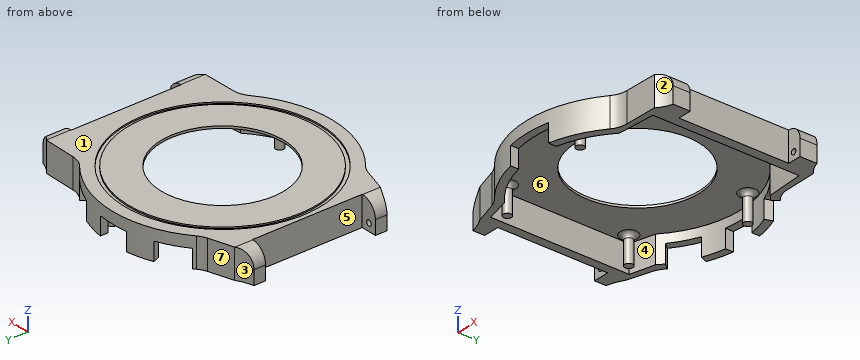
```python
from build123d import *

# Parameters (mm, degrees)
PAD_DEPTH       = 6.5
POCKET_DEPTH    = 6
SKETCH002_R     = 13.5
POCKET001_DEPTH = 1
SKETCH003_W     = 5.4
SKETCH003_H     = 6.5
PAD001_DEPTH    = 3
POCKET002_DEPTH = 10
SKETCH008_R     = 0.6
POCKET003_DEPTH = 2
SKETCH009_R     = 0.6
POCKET004_DEPTH = 2
FILLET_R        = 2.9
FILLET001_R     = 2.9
FILLET002_R     = 5
FILLET003_R     = 5
FILLET004_R     = 5
FILLET005_R     = 5
SKETCH010_W     = 3.95
SKETCH010_H     = 6.5
PAD002_DEPTH    = 3.5
POCKET005_DEPTH = 10
SKETCH012_R     = 0.6
POCKET006_DEPTH = 2
SKETCH013_R     = 0.6
POCKET007_DEPTH = 2
FILLET006_R     = 3.4
FILLET007_R     = 3.4
SKETCH014_R     = 21.6
SKETCH014_R_2   = 20.8
POCKET008_DEPTH = 0.3
SKETCH015_R     = 0.9
PAD003_DEPTH    = 6
FILLET008_R     = 1
POCKET009_DEPTH = 4
POCKET010_DEPTH = 4


with BuildPart() as part:
    # Sketch → Pad (new body)
    with BuildSketch(Plane.XY):
        with BuildLine():
            Line((-22.5019915649, 16), (-22.5019915649, -16))
            Line((-22.5019915649, -16), (-16.2858834578, -17.9))
            ThreePointArc((-16.2858834578, -17.9), (0.2206895736, -24.1989937004), (16.6096357576, -17.6))
            Line((16.6096357576, -17.6), (25.6083856708, -17.45))
            Line((25.6083856708, 17.45), (25.6083856708, -17.45))
            Line((16.6096357576, 17.6), (25.6083856708, 17.45))
            ThreePointArc((16.6096357576, 17.6), (0.2206895736, 24.1989937004), (-16.2858834578, 17.9))
            Line((-22.5019915649, 16), (-16.2858834578, 17.9))
        make_face()
    extrude(amount=PAD_DEPTH)

    # Sketch001 → Pocket (cut)
    with BuildSketch(Plane.XY):
        with BuildLine():
            Line((-15.2429491897, 16.55), (-20.5746937447, 15.2))
            Line((-20.5746937447, 15.2), (-20.5746937447, -15.2))
            Line((-20.5746937447, -15.2), (-15.2429491897, -16.55))
            ThreePointArc((-15.2429491897, -16.55), (0, -22.5), (15.2429491897, -16.55))
            Line((15.2429491897, -16.55), (23.5278752606, -16.05))
            Line((23.5278752606, 16.05), (23.5278752606, -16.05))
            Line((15.2429491897, 16.55), (23.5278752606, 16.05))
            ThreePointArc((15.2429491897, 16.55), (0, 22.5), (-15.2429491897, 16.55))
        make_face()
    extrude(amount=POCKET_DEPTH, mode=Mode.SUBTRACT)

    # Sketch002 (on Face19 of Pocket) → Pocket001 (cut)
    with BuildSketch(Plane(origin=(0, 0, 6), x_dir=(1, 0, 0), z_dir=(0, 0, -1))):
        Circle(SKETCH002_R)
    extrude(amount=-POCKET001_DEPTH, mode=Mode.SUBTRACT)

    # Sketch003 (on Face6 of Pocket001) → Pad001 (join)
    with BuildSketch(Plane.YZ.offset(25.6083856708)):
        with Locations((-14.75, 3.25)):
            Rectangle(SKETCH003_W, SKETCH003_H)
        with Locations((14.75, 3.25)):
            Rectangle(SKETCH003_W, SKETCH003_H)
    extrude(amount=PAD001_DEPTH)

    # Sketch006 → Pocket002 (cut)
    with BuildSketch(Plane.XY.offset(6.5)):
        with BuildLine():
            ThreePointArc((25.6083856708, 17.45), (27.0135397777, 16.4426436477), (28.6083856708, 15.775042373))
            Line((28.6083856708, 17.45), (28.6083856708, 15.775042373))
            Line((28.6083856708, 17.45), (25.6083856708, 17.45))
        make_face()
        with BuildLine():
            ThreePointArc((28.6083856708, -15.775042373), (27.0135397777, -16.4426436477), (25.6083856708, -17.45))
            Line((28.6083856708, -17.45), (25.6083856708, -17.45))
            Line((28.6083856708, -15.775042373), (28.6083856708, -17.45))
        make_face()
    extrude(amount=-POCKET002_DEPTH, mode=Mode.SUBTRACT)

    # Sketch008 (on Face27 of Pocket002) → Pocket003 (cut)
    with BuildSketch(Plane(origin=(0, -12.05, 0), x_dir=(-1, 0, 0), z_dir=(0, 1, 0))):
        with Locations((-26.9083856708, 1.7)):
            Circle(SKETCH008_R)
    extrude(amount=-POCKET003_DEPTH, mode=Mode.SUBTRACT)

    # Sketch009 (on Face26 of Pocket003) → Pocket004 (cut)
    with BuildSketch(Plane.XZ.offset(-12.05)):
        with Locations((26.9083856708, 1.7)):
            Circle(SKETCH009_R)
    extrude(amount=-POCKET004_DEPTH, mode=Mode.SUBTRACT)

    # Fillet
    fillet_edges = [part.edges().sort_by_distance(p)[0] for p in [
        (28.608386, -13.912521, 6.5),
    ]]
    fillet(fillet_edges, radius=FILLET_R)

    # Fillet001
    fillet001_edges = [part.edges().sort_by_distance(p)[0] for p in [
        (28.608386, 13.912521, 6.5),
    ]]
    fillet(fillet001_edges, radius=FILLET001_R)

    # Fillet002
    fillet002_edges = [part.edges().sort_by_distance(p)[0] for p in [
        (16.609636, -17.6, 3.25),
    ]]
    fillet(fillet002_edges, radius=FILLET002_R)

    # Fillet003
    fillet003_edges = [part.edges().sort_by_distance(p)[0] for p in [
        (16.609636, 17.6, 3.25),
    ]]
    fillet(fillet003_edges, radius=FILLET003_R)

    # Fillet004
    fillet004_edges = [part.edges().sort_by_distance(p)[0] for p in [
        (-16.285883, -17.9, 3.25),
    ]]
    fillet(fillet004_edges, radius=FILLET004_R)

    # Fillet005
    fillet005_edges = [part.edges().sort_by_distance(p)[0] for p in [
        (-16.285883, 17.9, 3.25),
    ]]
    fillet(fillet005_edges, radius=FILLET005_R)

    # Sketch010 (on Face4 of Fillet005) → Pad002 (join)
    with BuildSketch(Plane(origin=(-22.5019915649, 0, 0), x_dir=(0, -1, 0), z_dir=(-1, 0, 0))):
        with Locations((-14.025, 3.25)):
            Rectangle(SKETCH010_W, SKETCH010_H)
        with Locations((14.025, 3.25)):
            Rectangle(SKETCH010_W, SKETCH010_H)
    extrude(amount=PAD002_DEPTH)

    # Sketch011 (on Face6 of Pad002) → Pocket005 (cut)
    with BuildSketch(Plane.XY.offset(6.5)):
        with BuildLine():
            ThreePointArc((-26.0019915649, 14.6), (-24.1926075875, 15.1515400564), (-22.5019915649, 16))
            Line((-22.5019915649, 16), (-26.0019915649, 16))
            Line((-26.0019915649, 16), (-26.0019915649, 14.6))
        make_face()
        with BuildLine():
            ThreePointArc((-22.5019915649, -16), (-24.1926075875, -15.1515400564), (-26.0019915649, -14.6))
            Line((-26.0019915649, -14.6), (-26.0019915649, -16))
            Line((-26.0019915649, -16), (-22.5019915649, -16))
        make_face()
    extrude(amount=-POCKET005_DEPTH, mode=Mode.SUBTRACT)

    # Sketch012 (on Face23 of Pocket005) → Pocket006 (cut)
    with BuildSketch(Plane(origin=(0, -12.05, 0), x_dir=(-1, 0, 0), z_dir=(0, 1, 0))):
        with Locations((24.3019915649, 1.7)):
            Circle(SKETCH012_R)
    extrude(amount=-POCKET006_DEPTH, mode=Mode.SUBTRACT)

    # Sketch013 (on Face21 of Pocket006) → Pocket007 (cut)
    with BuildSketch(Plane.XZ.offset(-12.05)):
        with Locations((-24.3019915649, 1.7)):
            Circle(SKETCH013_R)
    extrude(amount=-POCKET007_DEPTH, mode=Mode.SUBTRACT)

    # Fillet006
    fillet006_edges = [part.edges().sort_by_distance(p)[0] for p in [
        (-26.001992, 13.325, 6.5),
    ]]
    fillet(fillet006_edges, radius=FILLET006_R)

    # Fillet007
    fillet007_edges = [part.edges().sort_by_distance(p)[0] for p in [
        (-26.001992, -13.325, 6.5),
    ]]
    fillet(fillet007_edges, radius=FILLET007_R)

    # Sketch014 (on Face4 of Fillet007) → Pocket008 (cut)
    with BuildSketch(Plane.XY.offset(6.5)):
        Circle(SKETCH014_R)
        Circle(SKETCH014_R_2, mode=Mode.SUBTRACT)
    extrude(amount=-POCKET008_DEPTH, mode=Mode.SUBTRACT)

    # Sketch015 (on Face55 of Pocket008) → Pad003 (join)
    with BuildSketch(Plane(origin=(0, 0, 6), x_dir=(1, 0, 0), z_dir=(0, 0, -1))):
        with Locations((-18.42, 13.32)):
            Circle(SKETCH015_R)
        with Locations((-18.42, -13.32)):
            Circle(SKETCH015_R)
        with Locations((7.27, 18.56)):
            Circle(SKETCH015_R)
        with Locations((5.37, -19.79)):
            Circle(SKETCH015_R)
    extrude(amount=PAD003_DEPTH)

    # Fillet008
    fillet008_edges = [part.edges().sort_by_distance(p)[0] for p in [
        (-19.32, -13.32, 6),
        (6.37, -18.56, 6),
        (-19.32, 13.32, 6),
        (4.47, 19.79, 6),
    ]]
    fillet(fillet008_edges, radius=FILLET008_R)

    # Sketch016 (on Face16 of Fillet008) → Pocket009 (cut)
    with BuildSketch(Plane(origin=(0, 0, 0), x_dir=(1, 0, 0), z_dir=(0, 0, -1))):
        with BuildLine():
            Line((-5, 23.6778377391), (-5, 21.9374109685))
            ThreePointArc((5, 21.9374109685), (0, 22.5), (-5, 21.9374109685))
            Line((5, 23.6778377391), (5, 21.9374109685))
            ThreePointArc((5, 23.6778377391), (0, 24.2), (-5, 23.6778377391))
        make_face()
    extrude(amount=-POCKET009_DEPTH, mode=Mode.SUBTRACT)

    # Sketch017 (on Face16 of Pocket009) → Pocket010 (cut)
    with BuildSketch(Plane(origin=(0, 0, 0), x_dir=(1, 0, 0), z_dir=(0, 0, -1))):
        with BuildLine():
            Line((-3.499984119, -22.2261132717), (-3.5, -23.9455632634))
            ThreePointArc((-3.5, -23.9455632634), (0, -24.2000019575), (3.5, -23.9455632634))
            Line((3.5000158811, -22.2261082701), (3.5, -23.9455632634))
            ThreePointArc((-3.499984119, -22.2261132717), (1.60767e-05, -22.5), (3.5000158811, -22.2261082701))
        make_face()
        with BuildLine():
            ThreePointArc((-13.9498796389, -17.6536358312), (-11.25, -19.4855715851), (-8.3135572795, -20.9077680626))
            Line((-8.3135572795, -20.9077680626), (-8.9416927184, -22.487466094))
            ThreePointArc((-15.0038705449, -18.987466094), (-12.1, -20.9578147716), (-8.9416927184, -22.487466094))
            Line((-13.9498796389, -17.6536358312), (-15.0038705449, -18.987466094))
        make_face()
        with BuildLine():
            ThreePointArc((8.3135572795, -20.9077680626), (11.25, -19.4855715851), (13.9498796389, -17.6536358312))
            Line((13.9498796389, -17.6536358312), (15.0038705449, -18.987466094))
            ThreePointArc((8.9416927184, -22.487466094), (12.1, -20.9578147716), (15.0038705449, -18.987466094))
            Line((8.3135572795, -20.9077680626), (8.9416927184, -22.487466094))
        make_face()
    extrude(amount=-POCKET010_DEPTH, mode=Mode.SUBTRACT)


solid = part.part
```
Design review of the part built by this model. Coordinates are the model's own, in mm. Face numbers are marked on the shaded views. A direction names the side the tool comes from. Give positions to 0.01 mm unless a question says otherwise; leave off trailing zeros. Order: outer loops, then holes, each group sorted by start corner. A loop starts at its lowest first (then second) coordinate and runs counter-clockwise, first axis right, second up. Notation, with made-up numbers: (-33.5, 63.5) -> (17.5, 63.5) arc R20 cw to (17.5, 89.5) -> close; hole circle Ø9 at (34.25, 44). An arc over 180 degrees is marked (long way). Write item = value, one per line. Start each with the question number.
(1) For the marked faces 5, 6 and 7, list the 3-axis set-ups (+Z, -Z, +X, -X, +Y, -Y) from which the entire face can be reached by the end or side of a thin tool; tool diameter is ignored.
(2) For pin 1 (1 mm diameter, centred on x = 26.91, z = 1.7, fed in from +Y); pin 2 (1.4 mm diameter, centred on y = -22.5, z = 1, fed in from -X); pin 3 (1.4 mm diameter, centred on x = -24.3, z = 1.7, fed in from -Y), all flat-tipped, find the tip position at first contact; note any pin that passes through.
(3) We need section C-C on x = -18.42. Write out the cut boundary in (y, z), plus the area to 3 significant figures.
(4) We need section B-B on x = -11. Write out the cut boundary in (y, z).
(5) We need section A-A on y = 0. Write out the cut boundary in (x, z).
(6) To check wall thickness, follow line 1 along Y through (x, z) = (0, 6.45); line 2 along X through (y, z) = (0, 4); line 3 along Z through (x, y) = (12, -18). State the ranges of each line that lie inside material, in increasing order.
(7) Mouldability with a two-part tool opening along Y and no side actions: class the marked faces 1, 2, 3 and 4 as +Y half, -Y half, draft (parallel to the pull), parting line (faces both ways), or undercut.
Numbers:
q1.face_5 = +Z, -Z, -X
q1.face_6 = -Z
q1.face_7 = +Z, -Z, -X, +Y
q2.pin_1 = 16.82
q2.pin_2 = -10.51
q2.pin_3 = -15.41
q3.outline = (-17.25, 0) -> (-15.75, 0) -> (-15.75, 6) -> (-15.22, 6) arc R1 cw to (-14.22, 5) -> (-14.22, 0) -> (-12.42, 0) -> (-12.42, 5) arc R1 cw to (-11.42, 6) -> (11.42, 6) arc R1 cw to (12.42, 5) -> (12.42, 0) -> (14.22, 0) -> (14.22, 5) arc R1 cw to (15.22, 6) -> (15.75, 6) -> (15.75, 0) -> (17.25, 0) -> (17.25, 6.5) -> (11.28, 6.5) -> (11.28, 6.2) -> (9.66, 6.2) -> (9.66, 6.5) -> (-9.66, 6.5) -> (-9.66, 6.2) -> (-11.28, 6.2) -> (-11.28, 6.5) -> (-17.25, 6.5) -> close
q3.area = 56.8 mm^2
q4.outline = (-21.56, 0) -> (-19.63, 0) -> (-19.63, 6) -> (-7.83, 6) -> (-7.83, 6.5) -> (-17.65, 6.5) -> (-17.65, 6.2) -> (-18.59, 6.2) -> (-18.59, 6.5) -> (-21.56, 6.5) -> close; (7.83, 6) -> (19.63, 6) -> (19.63, 4) -> (21.56, 4) -> (21.56, 6.5) -> (18.59, 6.5) -> (18.59, 6.2) -> (17.65, 6.2) -> (17.65, 6.5) -> (7.83, 6.5) -> close
q5.outline = (-22.5, 0) -> (-20.57, 0) -> (-20.57, 6) -> (-13.5, 6) -> (-13.5, 6.5) -> (-20.8, 6.5) -> (-20.8, 6.2) -> (-21.6, 6.2) -> (-21.6, 6.5) -> (-22.5, 6.5) -> close; (13.5, 6) -> (23.53, 6) -> (23.53, 0) -> (25.61, 0) -> (25.61, 6.5) -> (21.6, 6.5) -> (21.6, 6.2) -> (20.8, 6.2) -> (20.8, 6.5) -> (13.5, 6.5) -> close
q6.line_1 = -24.2 to -21.6, -20.8 to -13.5, 13.5 to 20.8, 21.6 to 24.2
q6.line_2 = -22.5 to -20.57, 23.53 to 25.61
q6.line_3 = 6 to 6.5
q7.face_1 = draft
q7.face_2 = -Y half
q7.face_3 = +Y half
q7.face_4 = undercut
